Input: part model. Units: mm. Frame: model coordinates. Coordinates: 2 decimals unless noted, no trailing zeros. Loops run counter-clockwise (first coordinate to the right, second up) from the corner with the lowest first, then second, coordinate; pieces in that order, holes last.
```python
from build123d import *

# Parameters (mm, degrees)
F0_W     = 609.6
F0_H     = 1219.2
F0_W_2   = 266.52658
F0_H_2   = 1011.554956
F1_DEPTH = 6.35
F2_R     = 5.08
F3_R     = 5.08


with BuildPart() as f1:
    # F0 (on Top) → F1 (new body)
    with BuildSketch(Plane.XY):
        Rectangle(F0_W, F0_H)
        Rectangle(F0_W_2, F0_H_2, mode=Mode.SUBTRACT)
    extrude(amount=F1_DEPTH)

    # F2
    f2_edges = [f1.edges().sort_by_distance(p)[0] for p in [
        (133.26329, 0, 6.35),
        (0, -505.777478, 6.35),
        (-133.26329, 0, 6.35),
        (0, 505.777478, 6.35),
    ]]
    fillet(f2_edges, radius=F2_R)

    # F3
    f3_edges = [f1.edges().sort_by_distance(p)[0] for p in [
        (-304.8, 0, 6.35),
        (304.8, 0, 6.35),
    ]]
    fillet(f3_edges, radius=F3_R)


solid = f1.part
```
Item 1: Section query B-B (y = -314.5). Output: boundary loops of the cut face in (x, z).
Result:
outline: (-304.8, 0) - (-133.26, 0) - (-133.26, 1.27) arc R5.08 ccw to (-138.34, 6.35) - (-299.72, 6.35) arc R5.08 ccw to (-304.8, 1.27) - close; (133.26, 0) - (304.8, 0) - (304.8, 1.27) arc R5.08 ccw to (299.72, 6.35) - (138.34, 6.35) arc R5.08 ccw to (133.26, 1.27) - close
Item 2: Contact query for a flat-ended pin moving along its axis: P1, Ø3, axis at y = -484.5, z = 4.5, coming from the +X side. Output: stop coordinate, or through.
Result:
P1: stops at x = 304.5
Item 3: Section query A-A (x = -64.5). Output: boundary loops of the cut face in (y, z), then the cut area to 3 significant figures.
Result:
outline: (-609.6, 0) - (-505.78, 0) - (-505.78, 1.27) arc R5.08 ccw to (-510.86, 6.35) - (-609.6, 6.35) - close; (505.78, 0) - (609.6, 0) - (609.6, 6.35) - (510.86, 6.35) arc R5.08 ccw to (505.78, 1.27) - close
area: 1,310 mm2
Item 4: Line query: L1, parallel to X at y = 449, z = 1; L2, parallel to Y at x = -2, z = 1.25; L3, parallel to Y at x = 125.5, z = 2.75. Output: solid intervals per line, ascending.
Result:
L1: x = -304.8 to -133.26, 133.26 to 304.8
L2: y = -609.6 to -505.78, 505.78 to 609.6
L3: y = -609.6 to -506, 506 to 609.6
Item 5: Section query C-C (z = 2.25). Output: boundary loops of the cut face in (x, y).
Result:
outline: (-304.7, -609.6) - (304.7, -609.6) - (304.7, 609.6) - (-304.7, 609.6) - close; hole (-133.36, -505.87) - (133.36, -505.87) - (133.36, 505.87) - (-133.36, 505.87) - close
